```python
from build123d import *

# Parameters (mm, degrees)
PAD008_DEPTH    = 8
CHAMFER001_SIZE = 7
SKETCH026_R     = 1.6
PAD009_DEPTH    = 13
SKETCH030_W     = 6
SKETCH030_H     = 6
POCKET014_DEPTH = 10
SKETCH031_R     = 1.25
POCKET015_DEPTH = 10.001
CHAMFER003_SIZE = 2
CHAMFER004_SIZE = 1


with BuildPart() as part:
    # Sketch025 → Pad008 (new body)
    with BuildSketch(Plane.XZ):
        with BuildLine():
            ThreePointArc((-12.901163, -1.6), (0, -13), (12.901163, -1.6))
            Line((3, -1.6), (12.901163, -1.6))
            Line((3, -2.8), (3, -1.6))
            ThreePointArc((-3, -2.8), (0, -5.8), (3, -2.8))
            Line((-3, -1.6), (-3, -2.8))
            Line((-3, -1.6), (-12.901163, -1.6))
        make_face()
    extrude(amount=PAD008_DEPTH)

    # Chamfer001
    chamfer001_edges = [part.edges().sort_by_distance(p)[0] for p in [
        (0, -8, -13),
    ]]
    chamfer(chamfer001_edges, length=CHAMFER001_SIZE)

    # Sketch026 → Pad009 (join)
    with BuildSketch(Plane.XY.offset(-1.6)):
        Polygon((24, 0), (-24, 0), (-24, 8.5), (-24, 10), (-13, 10), (-13, 4), (13, 4), (13, 10), (24, 10), (24, 8.5), align=None)
        with Locations((-20, 4.953278)):
            Circle(SKETCH026_R, mode=Mode.SUBTRACT)
        with Locations((20, 4.953278)):
            Circle(SKETCH026_R, mode=Mode.SUBTRACT)
    extrude(amount=-PAD009_DEPTH)

    # Sketch030 → Pocket014 (cut)
    with BuildSketch(Plane.XZ):
        with Locations((0, -3)):
            Rectangle(SKETCH030_W, SKETCH030_H)
    extrude(amount=-POCKET014_DEPTH, mode=Mode.SUBTRACT)

    # Sketch031 → Pocket015 (cut, through all)
    with BuildSketch(Plane.XZ):
        with Locations((-17, -10)):
            Circle(SKETCH031_R)
        with Locations((17, -10)):
            Circle(SKETCH031_R)
    extrude(amount=-POCKET015_DEPTH, mode=Mode.SUBTRACT)

    # Chamfer003
    chamfer003_edges = [part.edges().sort_by_distance(p)[0] for p in [
        (18.4, 4.953278, -14.6),
        (-21.6, 4.953278, -14.6),
    ]]
    chamfer(chamfer003_edges, length=CHAMFER003_SIZE)

    # Chamfer004
    chamfer004_edges = [part.edges().sort_by_distance(p)[0] for p in [
        (0, 0, -14.6),
    ]]
    chamfer(chamfer004_edges, length=CHAMFER004_SIZE)


solid = part.part
```
Check sheet for the modelled part. Datum: model origin and axes. Units: mm. A direction names the side the tool comes from. Coordinates: 2 decimals unless noted, no trailing zeros. Loops run counter-clockwise (first coordinate to the right, second up) from the corner with the lowest first, then second, coordinate; pieces in that order, holes last.
1) Gauge pin test, flat ends, axial feed: pin 1 (4 mm diameter, centred on x = -20, y = 4.95, fed in from -Z); pin 2 (2 mm diameter, centred on x = 12.5, z = -7.5, fed in from +Y); pin 3 (2 mm diameter, centred on x = -17, z = -10, fed in from -Y); pin 4 (4 mm diameter, centred on x = 1.5, z = -7, fed in from +Y). Record the tip position at first contact, or that the pin passes through.
2) Access from +Z, -Z, +X, -X, +Y, -Y to the whole of each face (thin tool, end or side, straight path). Record for faces 4 (the face through (0, 4, -8)), 5 (the face through (-3, -1, -2)), 6 (the face through (-5, 0, -13)).
3) Material ranges on probe 1 along X at (y, z) = (9.25, -8); probe 2 along Y at (x, z) = (-20, -4.5); probe 3 along X at (y, z) = (5.5, -3), recorded low to high.
4) Sectioned sample at B-B (x = -20). Record the boundary of the cut face in (y, z).
5) Sectioned sample at C-C (z = -10). Count the separate pieces of the cut face and the enclosed holes in it, and give its area (3 significant figures).
6) Release check for a two-part mould opening along X. For faces 1 (the face through (-13, 7, -8)), 2 (the face through (-1.3, -8, -5.7)), 3 (the face through (0, -6, -8)) record: released by +X, released by -X, zero draft, split by the parting line, or undercut.
7) Sectioned sample at A-A (x = 0). Record the boundary of the cut face in (y, z).
Check sheet entries:
1. pin 1: stops at z = -13
1. pin 2: stops at y = 10
1. pin 3: passes through
1. pin 4: stops at y = 4
2. face 4: +Z, -Z, +Y
2. face 5: +Z, +Y
2. face 6: -Z, -Y
3. probe 1: x = -24 to -13, 13 to 24
3. probe 2: y = 0 to 3.35, 6.55 to 10
3. probe 3: x = -24 to -21.5, -18.5 to -13, 13 to 18.5, 21.5 to 24
4. outline: (0, -13.6) - (1, -14.6) - (1.35, -14.6) - (3.35, -12.6) - (3.35, -1.6) - (0, -1.6) - close; (6.55, -12.6) - (8.55, -14.6) - (10, -14.6) - (10, -1.6) - (6.55, -1.6) - close
5. separate pieces: 3
5. enclosed holes: 2
5. area: 307 mm2
6. face 1: undercut
6. face 2: zero draft
6. face 3: split by the parting line
7. outline: (-8, -6) - (-1, -13) - (0, -13) - (0, -13.6) - (1, -14.6) - (4, -14.6) - (4, -6) - (0, -6) - (0, -5.8) - (-8, -5.8) - close
